```python
from build123d import *

# Parameters (mm, degrees)
SKETCH_8_R      = 1.25
SKETCH_8_R_2    = 3
SKETCH_8_R_3    = 1
EXTRUDE_1_DEPTH = 2


with BuildPart() as part:
    # 草圖8 → 填料-伸長1 (new body)
    with BuildSketch(Plane.XY):
        with BuildLine():
            Line((-23.40478598, 11.861352689), (-23.40478598, 9.861352689))
            ThreePointArc((-23.40478598, 9.861352689), (-22.40478598, 8.861352689), (-23.40478598, 7.861352689))
            Line((-23.40478598, 7.861352689), (-25.40478598, 7.861352689))
            Line((-25.40478598, 7.861352689), (-25.40478598, 3.861352689))
            Line((-25.40478598, 3.861352689), (-23.40478598, 3.861352689))
            ThreePointArc((-23.40478598, 3.861352689), (-22.40478598, 2.861352689), (-23.40478598, 1.861352689))
            Line((-23.40478598, 1.861352689), (-23.40478598, -2.138647311))
            ThreePointArc((-23.40478598, -2.138647311), (-22.40478598, -3.138647311), (-23.40478598, -4.138647311))
            Line((-23.40478598, -4.138647311), (-25.40478598, -4.138647311))
            Line((-25.40478598, -4.138647311), (-25.40478598, -8.138647311))
            Line((-25.40478598, -8.138647311), (-23.40478598, -8.138647311))
            ThreePointArc((-23.40478598, -8.138647311), (-22.40478598, -9.138647311), (-23.40478598, -10.138647311))
            Line((-23.40478598, -10.138647311), (-23.40478598, -12.138647311))
            Line((-23.40478598, -12.138647311), (-3.40478598, -12.138647311))
            ThreePointArc((-3.40478598, -12.138647311), (8.59521402, -0.138647311), (-3.40478598, 11.861352689))
            Line((-3.40478598, 11.861352689), (-23.40478598, 11.861352689))
        make_face()
        with Locations((-3.40478598, 6.861352689)):
            Circle(SKETCH_8_R, mode=Mode.SUBTRACT)
        with Locations((1.544961489, 4.811100157)):
            Circle(SKETCH_8_R, mode=Mode.SUBTRACT)
        with Locations((-3.40478598, -0.138647311)):
            Circle(SKETCH_8_R_2, mode=Mode.SUBTRACT)
        with Locations((3.59521402, -0.138647311)):
            Circle(SKETCH_8_R, mode=Mode.SUBTRACT)
        with Locations((1.544961489, -5.08839478)):
            Circle(SKETCH_8_R, mode=Mode.SUBTRACT)
        with Locations((-3.40478598, -7.138647311)):
            Circle(SKETCH_8_R, mode=Mode.SUBTRACT)
        with Locations((-8.354533448, -5.08839478)):
            Circle(SKETCH_8_R, mode=Mode.SUBTRACT)
        with Locations((-10.40478598, -0.138647311)):
            Circle(SKETCH_8_R, mode=Mode.SUBTRACT)
        with Locations((-8.354533448, 4.811100157)):
            Circle(SKETCH_8_R, mode=Mode.SUBTRACT)
        with Locations((-21.40478598, 5.861352689)):
            Circle(SKETCH_8_R_3, mode=Mode.SUBTRACT)
        with Locations((-21.40478598, -6.138647311)):
            Circle(SKETCH_8_R_3, mode=Mode.SUBTRACT)
    extrude(amount=EXTRUDE_1_DEPTH)


solid = part.part
```
CAD build for the part. Positions are in the model's coordinates, mm. A direction names the side the tool comes from. Round coordinates to 2 decimals unless told otherwise and drop trailing zeros. Write each loop counter-clockwise with the first axis right and the second up, starting at its lowest first coordinate (ties: lowest second). Pieces come first, ordered by that corner, then holes. Notation, with made-up numbers: (38, -14.75) - (87, -14.75) arc R24 ccw to (87, 7.25) - close; hole circle Ø6 at (34.25, 63). An arc over 180 degrees is marked (long way). Return JSON: item names as keys, results as strings. Group by question number.
Item 1: Mould opens along Y. For faces 4 (the face through (-22.405, -9.117, 0.986)), 5 (the face through (-13, 11.861, 1)), 6 (the face through (8.592, -0.403, 0.986)) say: +Y half, -Y half, draft (parallel to the pull), parting line (faces both ways), or undercut.
Item 2: Band-saw the part on B-B on x = -2.5. List the corners of the cut face in (y, z), plus the area to 3 significant figures.
Item 3: Band-saw the part on C-C on z = 1.4. State how many separate pieces and enclosed holes the cut face has, plus the area to 3 significant figures.
Item 4: Band-saw the part on D-D on y = -3.5. List the corners of the cut face in (x, z), plus the area to 3 significant figures.
Item 5: Band-saw the part on A-A on y = 0.75. List the corners of the cut face in (x, z).
Item 6: 3-axis set-ups, long thin cutter, end or side, ignore diameter. For faces 1 (the face through (-23.405, 0, 1)), 2 (the face through (-23.405, -11, 1)), 3 (the face through (-8.63, 3.59, 0.99)): which of +Z, -Z, +X, -X, +Y, -Y reach the whole face in a straight line?
Item 7: Probe probe 1 along X at (y, z) = (4.75, 0.55); probe 2 along X at (y, z) = (5.75, 0.9); probe 3 along Y at (x, z) = (-4, 1.8). List the from-to ranges inside material, lowest first.
Item 8: Flat gauge pin, fed straight in: pin 1 Ø1 at (x, z) = (-25, 1) entering from +Y. Where does the tip first touch, or does it go through?
Resolved:
{
 "1": {"face 4": "undercut", "face 5": "+Y half", "face 6": "parting line"},
 "2": {"outline": "(-12.1, 0) - (-8, 0) - (-8, 2) - (-12.1, 2) - close; (-6.28, 0) - (-3, 0) - (-3, 2) - (-6.28, 2) - close; (2.72, 0) - (6, 0) - (6, 2) - (2.72, 2) - close; (7.72, 0) - (11.83, 0) - (11.83, 2) - (7.72, 2) - close", "area": "29.5 mm²"},
 "3": {"separate pieces": "1", "enclosed holes": "11", "area": "642 mm²"},
 "4": {"outline": "(-22.47, 0) - (8.11, 0) - (8.11, 2) - (-22.47, 2) - close", "area": "61.2 mm²"},
 "5": {"outline": "(-23.4, 0) - (-11.28, 0) - (-11.28, 2) - (-23.4, 2) - close; (-9.53, 0) - (-6.27, 0) - (-6.27, 2) - (-9.53, 2) - close; (-0.54, 0) - (2.72, 0) - (2.72, 2) - (-0.54, 2) - close; (4.47, 0) - (8.56, 0) - (8.56, 2) - (4.47, 2) - close"},
 "6": {"face 1": "+Z, -Z, -X", "face 2": "+Z, -Z, -X, -Y", "face 3": "+Z, -Z"},
 "7": {"probe 1": "x = -25.4 to -9.6, -7.11 to 0.3, 2.79 to 7.55", "probe 2": "x = -25.4 to -22.4, -20.41 to -9.18, -7.53 to -3.98, -2.83 to 0.72, 2.37 to 7.05", "probe 3": "y = -12.14 to -8.24, -6.04 to -3.08, 2.8 to 5.76, 7.96 to 11.86"},
 "8": {"pin 1": "stops at y = 7.86"}
}
